```python
from build123d import *

# Parameters (mm, degrees)
SKETCH1_R           = 9.525
SKETCH1_R_2         = 8.73125
BOSS_EXTRUDE1_DEPTH = 12.7
BOSS_EXTRUDE2_DEPTH = 6.35
SKETCH4_R           = 8.73125
CUT_EXTRUDE1_DEPTH  = 37.153197474


with BuildPart() as part:
    # Sketch1 → Boss-Extrude1 (new body)
    with BuildSketch(Plane.XY):
        Circle(SKETCH1_R)
        Circle(SKETCH1_R_2, mode=Mode.SUBTRACT)
    extrude(amount=BOSS_EXTRUDE1_DEPTH)

    # Sketch2 → Boss-Extrude2 (add)
    with BuildSketch(Plane(origin=(0, 0, 0), x_dir=(-1, 0, 0), z_dir=(0, 0, -1))):
        Polygon((-10.484370366, -7.397850118), (1.164540953, -12.778656138), (11.648911318, -5.38080602), (10.484370366, 7.397850118), (-1.164540953, 12.778656138), (-11.648911318, 5.38080602), align=None)
    extrude(amount=BOSS_EXTRUDE2_DEPTH)

    # Sketch3 → Revolve1 (revolve)
    with BuildSketch(Plane(origin=(0, 0, 0), x_dir=(0, 0, -1), z_dir=(1, 0, 0)), mode=Mode.PRIVATE) as revolve1_sk:
        Polygon((6.35, 8.73125), (19.05, 8.73125), (19.05, 10.05294024), (17.470288197, 11.034529182), (17.470288197, 9.882889591), (15.616906831, 11.034529182), (15.616906831, 9.882889591), (13.763525465, 11.034529182), (13.763525465, 9.882889591), (11.910144098, 11.034529182), (11.910144098, 9.882889591), (10.056762732, 11.034529182), (10.056762732, 9.882889591), (8.203381366, 11.034529182), (8.203381366, 9.882889591), (6.35, 11.034529182), align=None)
    revolve(revolve1_sk.sketch.rotate(Axis((0, 0, 0), (0, 0, -1)), 90), axis=Axis((0, 0, 0), (0, 0, -1)))

    # Sketch4 → Cut-Extrude1 (cut, through all)
    with BuildSketch(Plane.XY.offset(12.7)):
        Circle(SKETCH4_R)
    extrude(amount=-CUT_EXTRUDE1_DEPTH, mode=Mode.SUBTRACT)


solid = part.part
```
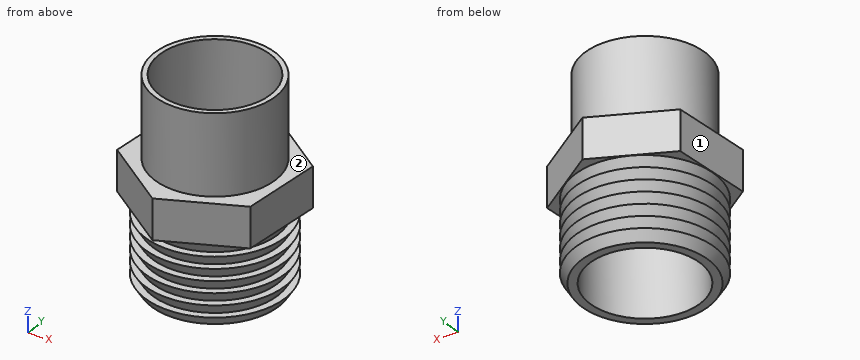
Can you work these out from the model? Positions are in its coordinate system, mm. Face numbers are marked on the shaded views. A direction names the side the tool comes from. Give positions to 0.01 mm unless a question says otherwise; leave off trailing zeros. One line per item, written item: value.
Q1. Please list where these lines run through material, in increasing order: line 1 (Y direction, x = 0, z = 10) (3 decimals); line 2 (X direction, y = -0.5, z = -3); line 3 (X direction, y = 6.25, z = 4). Write a range as [from, to].
Results found:
line 1: y = [-9.525, -8.731], [8.731, 9.525]
line 2: x = [-11.2, -8.72], [8.72, 11.11]
line 3: x = [-7.19, -6.1], [6.1, 7.19]
Q2. For P1, Ø1.5, axis at x = -4.5, z = -15.5, coming from the -Y side; P2, Ø6, axis at x = 3.5, z = 8.5, coming from the -Y side; P3, Ø1.5, axis at x = -6.5, y = 4, coming from the -Z side; P4, Ø1, axis at y = 8.5, z = -8, coming from the +X side, each with a flat end and sliding along its axis, tell me the tip position at first contact or that it passes through.
Results found:
P1: stops at y = -10.37
P2: stops at y = -9.51
P3: passes through
P4: stops at x = 7.55
Q3. Which directions (+Z, -Z, +X, -X, +Y, -Y) give clear straight access to the entire face, cutting with the end or side of a thin tool? Please do the marked faces 1 and 2.
Results found:
face 1: +Z, -Z, -X, +Y
face 2: +Z
